from build123d import *

# Parameters (mm, degrees)
SKETCH1_W           = 500
SKETCH1_H           = 360
BOSS_EXTRUDE1_DEPTH = 260
SKETCH2_W           = 90
SKETCH2_H           = 360
BOSS_EXTRUDE3_DEPTH = 70
SKETCH3_W           = 300
SKETCH3_H           = 80
BOSS_EXTRUDE4_DEPTH = 110
SKETCH4_W           = 180
SKETCH4_H           = 200
BOSS_EXTRUDE5_DEPTH = 220


with BuildPart() as part:
    # Sketch1 → Boss-Extrude1 (new body)
    with BuildSketch(Plane(origin=(0, 0, 0), x_dir=(1, 0, 0), z_dir=(0, 1, 0))):
        with Locations((250, 180)):
            Rectangle(SKETCH1_W, SKETCH1_H)
    extrude(amount=-BOSS_EXTRUDE1_DEPTH)

    # Sketch2 → Boss-Extrude3 (add)
    with BuildSketch(Plane(origin=(0, 0, 0), x_dir=(1, 0, 0), z_dir=(0, 1, 0))):
        with Locations((45, 180)):
            Rectangle(SKETCH2_W, SKETCH2_H)
    extrude(amount=BOSS_EXTRUDE3_DEPTH)

    # Sketch3 → Boss-Extrude4 (add)
    with BuildSketch(Plane(origin=(0, 0, 0), x_dir=(1, 0, 0), z_dir=(0, 1, 0))):
        with Locations((240, 320)):
            Rectangle(SKETCH3_W, SKETCH3_H)
        with Locations((240, 40)):
            Rectangle(SKETCH3_W, SKETCH3_H)
    extrude(amount=BOSS_EXTRUDE4_DEPTH)

    # Sketch4 → Boss-Extrude5 (add)
    with BuildSketch(Plane(origin=(0, 0, 0), x_dir=(1, 0, 0), z_dir=(0, 1, 0))):
        with Locations((410, 180)):
            Rectangle(SKETCH4_W, SKETCH4_H)
    extrude(amount=BOSS_EXTRUDE5_DEPTH)


solid = part.part
Read the model definition and answer for the solid it produces. Units are mm, in the model's axes. A direction names the side the tool comes from. Round coordinates to 2 decimals unless told otherwise and drop trailing zeros. Write each loop counter-clockwise with the first axis right and the second up, starting at its lowest first coordinate (ties: lowest second). Pieces come first, ordered by that corner, then holes. Notation, with made-up numbers: M 70.5,52 L 117.5,52 A8 cw 117.5,62 Z; hole C -23.75,4 d3. An arc over 180 degrees is marked long. Use a Markdown table: item, result.
1) A tool of negligible diameter and unlimited length cuts with its end or side. For faces 5 (the flat face through (203, 0, -181)), 6 (the flat face through (390, 54, -319)), 7 (the flat face through (238, 110, -41)), 8 (the flat face through (44, 70, -183)), 9 (the flat face through (238, 110, -321)), from which of +Z, -Z, +X, -X, +Y, -Y can it reach the whole face along a straight path? Write none if from no direction.
Answers follow:
| item | result |
|---|---|
| face 5 | +Y |
| face 6 | -Z, +X, +Y |
| face 7 | +Z, +X, -X, +Y |
| face 8 | +Z, -Z, -X, +Y |
| face 9 | -Z, +X, -X, +Y |
2) The part is cut by section C-C (z = -121). Write down the section's boundary in (x, y).
Answers follow:
| item | result |
|---|---|
| outline | M 0,-260 L 500,-260 L 500,220 L 320,220 L 320,0 L 90,0 L 90,70 L 0,70 Z |
3) Flat-ended cylindrical pins translate along their axes: pin 1 (24 mm diameter, centred on y = 49.5, z = -312.5, fed in from +X); pin 2 (24 mm diameter, centred on x = 196.5, z = -59, fed in from +Y); pin 3 (3 mm diameter, centred on x = 251, z = -208.5, fed in from +Y). Find the tip coordinate at first contact, or state that the pin passes through.
Answers follow:
| item | result |
|---|---|
| pin 1 | stops at x = 390 |
| pin 2 | stops at y = 110 |
| pin 3 | stops at y = 0 |
4) For a pull along Z with two mould halves and no side action, classify faces 1 (the flat face through (247, -78, -360)), 2 (the flat face through (247, -78, 0)), 3 (the flat face through (320, 108, -179)), 4 (the flat face through (444, 0, -41)) as pulls with the +Z half, pulls with the -Z half, needs draft (parallel to the pull), parting line crosses it, or undercut.
Answers follow:
| item | result |
|---|---|
| face 1 | pulls with the -Z half |
| face 2 | pulls with the +Z half |
| face 3 | undercut |
| face 4 | needs draft |
5) The part is cut by section B-B (x = 379). Write down the section's boundary in (y, z), plus the area to 3 significant figures.
Answers follow:
| item | result |
|---|---|
| outline | M -260,-360 L 110,-360 L 110,-280 L 220,-280 L 220,-80 L 110,-80 L 110,0 L -260,0 Z |
| area | 155,000 mm2 |
6) Straight lines are drawn through the part: line 1 along X through (y, z) = (9, -116); line 2 along Y through (x, z) = (308, -231.5); line 3 along X through (y, z) = (108.5, -156). For each, find the intervals that lie inside material, in ascending order. Write a range as [from, to].
Answers follow:
| item | result |
|---|---|
| line 1 | x = [0, 90], [320, 500] |
| line 2 | y = [-260, 0] |
| line 3 | x = [320, 500] |
7) The part is cut by section A-A (y = 26). Write down the section's boundary in (x, z), plus the area to 3 significant figures.
Answers follow:
| item | result |
|---|---|
| outline | M 0,-360 L 390,-360 L 390,-280 L 500,-280 L 500,-80 L 390,-80 L 390,0 L 0,0 Z; hole M 90,-280 L 320,-280 L 320,-80 L 90,-80 Z |
| area | 116,000 mm2 |
